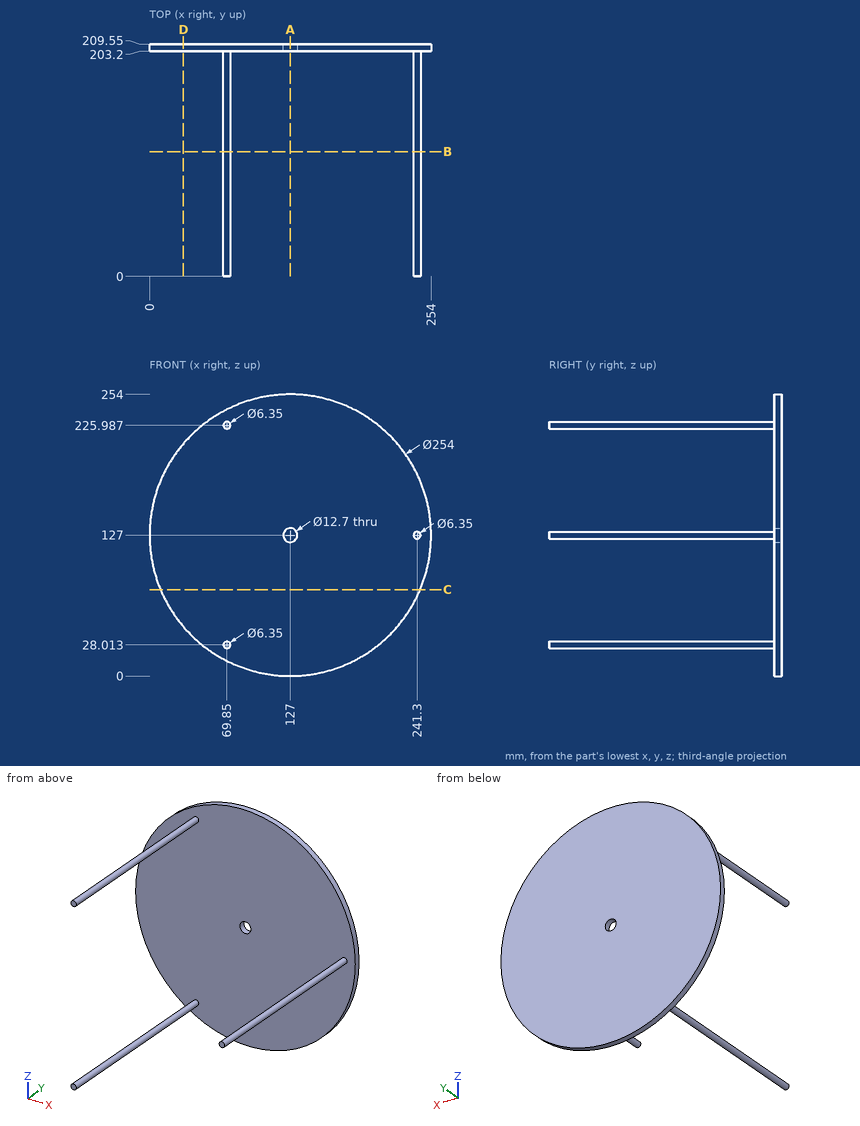
Source: three-view drawing plus pictorial views. Frame: mm from the lowest corner of the part. Round coordinates to 2 decimals unless told otherwise and drop trailing zeros. Loops run counter-clockwise (first coordinate to the right, second up) from the corner with the lowest first, then second, coordinate; pieces in that order, holes last.
Item 1: Section B-B, the plane y = 112.5. State how many separate pieces and enclosed holes the cut face has, plus the area to 3 significant figures.
Checked values:
separate pieces: 3
enclosed holes: 0
area: 95.0 mm2
Item 2: Section C-C, the plane z = 78. Output: boundary loops of the cut face in (x, y).
Checked values:
outline: (9.83, 203.2) - (244.17, 203.2) - (244.17, 209.55) - (9.83, 209.55) - close
Item 3: Line query: L1, parallel to Z at x = 127, y = 207; L2, parallel to Y at x = 98.5, z = 15.5; L3, parallel to X at y = 130, z = 224. Output: solid intervals per line, ascending.
Checked values:
L1: z = 0 to 120.65, 133.35 to 254
L2: y = 203.2 to 209.55
L3: x = 67.37 to 72.33
Item 4: Contact query for a flat-ended pin moving along its axis: P1, Ø20.5, axis at x = 127, z = 127, coming from the -Y side. Output: stop coordinate, or through.
Checked values:
P1: stops at y = 203.2
Item 5: Section A-A, the plane x = 127. Output: boundary loops of the cut face in (y, z), plus the area to 3 significant figures.
Checked values:
outline: (203.2, 0) - (209.55, 0) - (209.55, 120.65) - (203.2, 120.65) - close; (203.2, 133.35) - (209.55, 133.35) - (209.55, 254) - (203.2, 254) - close
area: 1,530 mm2
Item 6: Section D-D, the plane x = 30.5. Output: boundary loops of the cut face in (y, z).
Checked values:
outline: (203.2, 44.44) - (209.55, 44.44) - (209.55, 209.56) - (203.2, 209.56) - close
